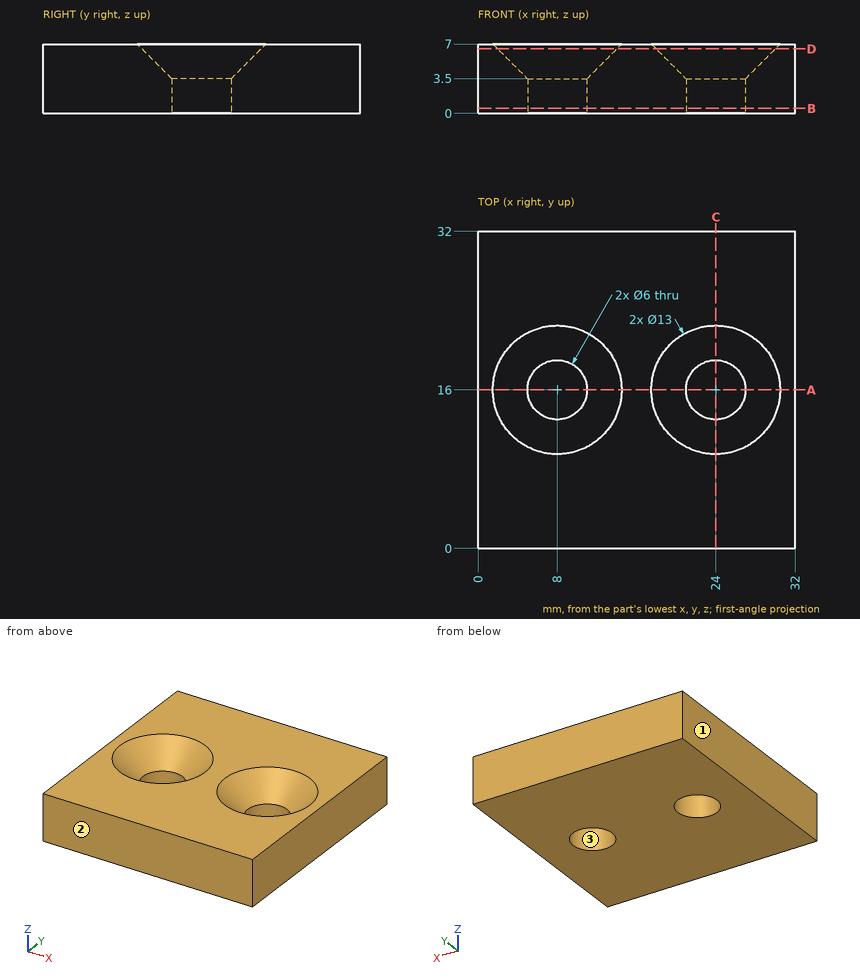
Design review of the part shown in the three views and the two pictorial views. Dimensions are in mm from the part's minimum x, y and z. Coordinates: 2 decimals unless noted, no trailing zeros. Order: outer loops, then holes, each group sorted by start corner. A loop starts at its lowest first (then second) coordinate and runs counter-clockwise, first axis right, second up.
1) Take a section at A-A, the plane y = 16. Give the boundary of the cut face in (x, z), and give its area (4 significant figures).
2) Mouldability with a two-part tool opening along X and no side actions: class the marked faces 1, 2 and 3 as +X half, -X half, draft (parallel to the pull), parting line (faces both ways), or undercut.
3) Take a section at D-D, the plane z = 6.5. Give the boundary of the cut face in (x, y).
4) Take a section at B-B, the plane z = 0.5. Give the boundary of the cut face in (x, y), and give its area (3 significant figures).
5) Clearance check with flat-ended pins moving along their axes: pin 1 (9.5 mm diameter, centred on x = 8, y = 16, fed in from +Z); pin 2 (1 mm diameter, centred on x = 19.5, y = 17, fed in from +Z). State where each tip first meets the part, or that it passes through.
6) Take a section at C-C, the plane x = 24. Give the boundary of the cut face in (y, z).
7) Wall thickness on line 1 along X through (y, z) = (16, 1.1); line 2 along Y through (x, z) = (8, 2.4); line 3 along X through (y, z) = (16.5, 5): over which ranges is each line inside the solid? List them lowest first.
Returned:
1. outline: (0, 0) - (5, 0) - (5, 3.5) - (1.5, 7) - (0, 7) - close; (11, 0) - (21, 0) - (21, 3.5) - (17.5, 7) - (14.5, 7) - (11, 3.5) - close; (27, 0) - (32, 0) - (32, 7) - (30.5, 7) - (27, 3.5) - close
1. area: 115.5 mm2
2. face 1: -X half
2. face 2: draft
2. face 3: undercut
3. outline: (0, 0) - (32, 0) - (32, 32) - (0, 32) - close; hole circle Ø12 at (8, 16); hole circle Ø12 at (24, 16)
4. outline: (0, 0) - (32, 0) - (32, 32) - (0, 32) - close; hole circle Ø6 at (8, 16); hole circle Ø6 at (24, 16)
4. area: 967 mm2
5. pin 1: stops at z = 5.25
5. pin 2: stops at z = 5.61
6. outline: (0, 0) - (13, 0) - (13, 3.5) - (9.5, 7) - (0, 7) - close; (19, 0) - (32, 0) - (32, 7) - (22.5, 7) - (19, 3.5) - close
7. line 1: x = 0 to 5, 11 to 21, 27 to 32
7. line 2: y = 0 to 13, 19 to 32
7. line 3: x = 0 to 3.53, 12.47 to 19.53, 28.47 to 32
